Geometry: final body of the model. Coordinates: model frame, mm. A direction names the side the tool comes from. Round coordinates to 2 decimals unless told otherwise and drop trailing zeros. Loops run counter-clockwise (first coordinate to the right, second up) from the corner with the lowest first, then second, coordinate; pieces in that order, holes last. Notation, with made-up numbers: (74, -21) - (133, -21) arc R12 ccw to (133, -3) - close; hole circle Ø3 at (40, -5.5). An arc over 180 degrees is marked (long way). Return JSON: item names as keys, results as strings. Group by question number.
1. Material intervals for probe 1 along Y at (x, z) = (24, 189); probe 2 along Z at (x, y) = (10, -16); probe 3 along X at (y, z) = (-22.5, 142.5), sorted ascending.
2. Draft query along Z for faces 4 (the face through (27, -23, 200)), 5 (the face through (17.5, -23, 26)), 6 (the face through (30, 13, 124)). Return one class per face: +Z half, -Z half, draft (parallel to the pull), parting line (faces both ways), or undercut.
3. First-contact query: pin 1 Ø8 at (x, y) = (23, -10) entering from -Z; pin 2 Ø8 at (x, y) = (-19.5, -15.5) entering from +Z; pin 3 Ø22 at (y, z) = (22.5, 167.5) entering from -X. Flat tips, straight axial feed; report the tip coordinate or a pass-through.
4. Section B-B on x = 10.5. Return loops of the section in (y, z), and give its area (3 significant figures).
5. Set-up query: faces 1 (the face through (17.5, -23, 151)), 2 (the face through (17.5, 23, 26)), 3 (the face through (27.5, 0, 49)). Return all of +Z, -Z, +X, -X, +Y, -Y with unobstructed straight access to the full face (end or side cutting, diameter ignored); none if empty.
6. Section A-A on z = 135. Return loops of the section in (x, y), and give its area (3 significant figures).
7. Section D-D on z = 76.5. Return loops of the section in (x, y), and give its area (3 significant figures).
8. Section C-C on y = 21.5. Return loops of the section in (x, z).
Autodesk Inventor part; units mm, degrees
ref_plane "YZ Plane" through (0, 0, 0) normal (1, 0, 0) x (0, 1, 0)
ref_plane "XZ Plane" through (0, 0, 0) normal (0, 1, 0) x (-1, 0, 0)
ref_plane "XY Plane" through (0, 0, 0) normal (0, 0, 1) x (1, 0, 0)
sketch "Sketch1" plane through (0, 0, 0) normal (0, 0, 1) x (1, 0, 0)
  line L0 (27.5, -33) -> (-27.5, -33)
  line L1 (-27.5, -33) -> (-27.5, 33)
  line L2 (-27.5, 33) -> (27.5, 33)
  line L3 (27.5, 33) -> (27.5, -33)
  line L4 (0, 0) -> (0, 15.9599)
  line L5 (0, 0) -> (14.573, 0)
  point P0 (0, 33)
  point P1 (27.5, 0)
  dimension "d0" = 55
  dimension "d1" = 66
extrude "Extrusion1" add sketch "Sketch1" along normal blind 100
sketch "Sketch2" plane through (-27.5, 33, 0) normal (0, 1, 0) x (1, 0, 0)
  circle A0 centre (38, -26) radius 8
  circle A1 centre (38, -26) radius 8
  point P0 (27.5, 0)
extrude "Extrusion2" cut sketch "Sketch2" against normal through all
sketch "Sketch3" plane through (27.5, -33, 0) normal (1, 0, 0) x (0, 0, -1)
  line L0 (0, 0) -> (-200, 0)
  line L1 (-200, 0) -> (-200, 20)
  line L2 (-200, 20) -> (0, 20)
  line L3 (0, 20) -> (0, 0)
  line L4 (0, 66) -> (-200, 66)
  line L5 (-200, 66) -> (-200, 46)
  line L6 (-200, 46) -> (0, 46)
  line L7 (0, 46) -> (0, 66)
  point P0 (0, 33)
  dimension "d6" = 200
  dimension "d7" = 20
  dimension "d8" = 200
  dimension "d9" = 20
extrude "Extrusion3" add sketch "Sketch3" along normal mid plane 20
properties part number "Support" material "Wood (Oak)"
Taken from the geometry:
{
 "1": {"probe 1": "-33 to -13, 13 to 33", "probe 2": "0 to 18.02, 33.98 to 100", "probe 3": "17.5 to 37.5"},
 "2": {"face 4": "+Z half", "face 5": "undercut", "face 6": "draft"},
 "3": {"pin 1": "z = 0", "pin 2": "z = 100", "pin 3": "x = 17.5"},
 "4": {"outline": "(-33, 0) - (33, 0) - (33, 18) - (-33, 18) - close; (-33, 34) - (33, 34) - (33, 100) - (-33, 100) - close", "area": "5,540 mm2"},
 "5": {"face 1": "+Z, -X, +Y, -Y", "face 2": "+Y, -Y", "face 3": "+Z, -Z, +X"},
 "6": {"outline": "(17.5, -33) - (37.5, -33) - (37.5, -13) - (17.5, -13) - close; (17.5, 13) - (37.5, 13) - (37.5, 33) - (17.5, 33) - close", "area": "800 mm2"},
 "7": {"outline": "(-27.5, -33) - (37.5, -33) - (37.5, -13) - (27.5, -13) - (27.5, 13) - (37.5, 13) - (37.5, 33) - (-27.5, 33) - close", "area": "4,030 mm2"},
 "8": {"outline": "(-27.5, 0) - (37.5, 0) - (37.5, 200) - (17.5, 200) - (17.5, 100) - (-27.5, 100) - close; hole (17.5, 22.13) - (17.5, 29.87) arc R8 ccw (long way) to start"}
}
